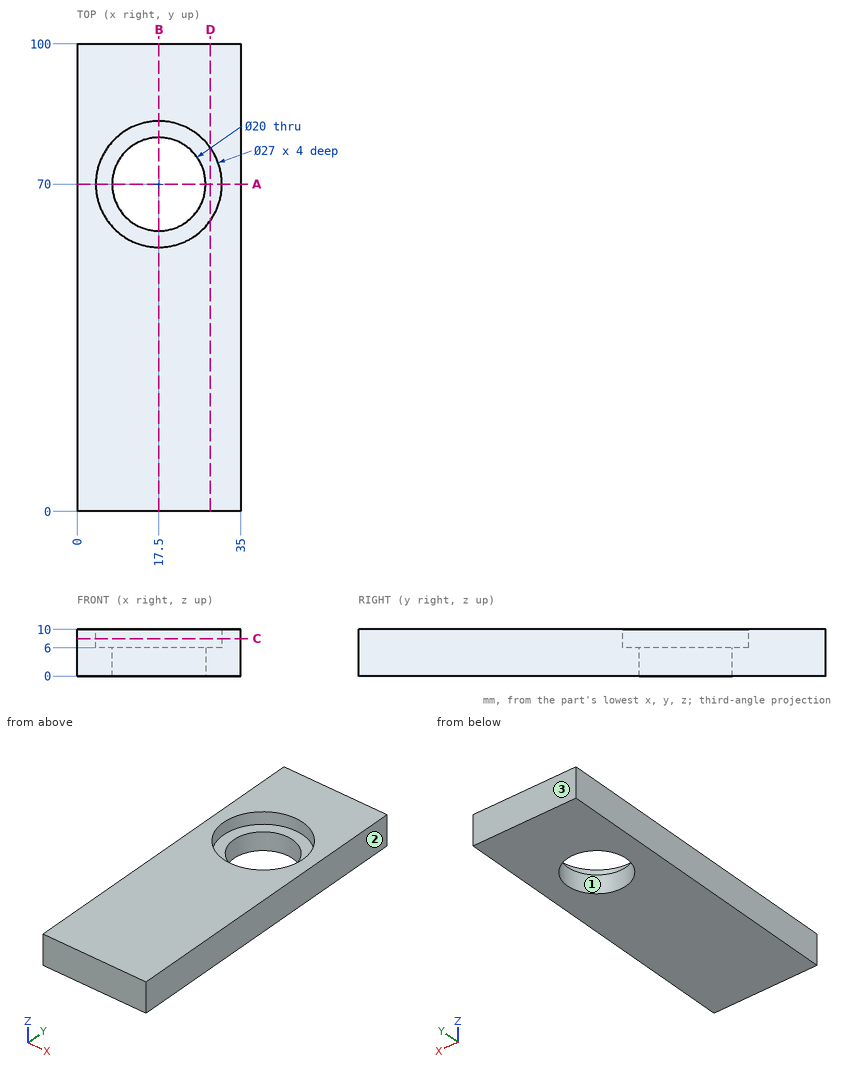
For this review, use the dimensioned drawing (mm, ordinates from the lowest corner) and the shaded views. Round coordinates to 2 decimals unless told otherwise and drop trailing zeros. Write each loop counter-clockwise with the first axis right and the second up, starting at its lowest first coordinate (ties: lowest second). Pieces come first, ordered by that corner, then holes. Notation, with made-up numbers: M 29.5,-33.5 L 82.5,-33.5 A11 cw 82.5,-27.5 Z; hole C 30.25,-20.5 d10. An arc over 180 degrees is marked long. Answer as CSV lines item,"result". Start each with the question number.
Q1. Consider section D-D, the plane x = 28.5. Give the boundary of the cut face in (y, z), then the cut area to 3 significant figures.
Q2. The part is to be moulded in two halves that separate along Y. For the marked faces 1, 2 and 3, say which applies: +Y half, -Y half, draft (parallel to the pull), parting line (faces both ways), or undercut.
Q3. Consider section B-B, the plane x = 17.5. Give the boundary of the cut face in (y, z).
Q4. Wall thickness on line 1 along Y through (x, z) = (17.5, 4); line 2 along Y through (x, z) = (17.5, 8.85); line 3 along Z through (x, y) = (4.5, 72.5): over which ranges is each line inside the solid? List them lowest first.
Q5. Consider section C-C, the plane z = 8. Give the boundary of the cut face in (x, y).
Q6. Consider section A-A, the plane y = 70. Give the boundary of the cut face in (x, z).
Result set:
1,outline,"M 0,0 L 100,0 L 100,10 L 77.83,10 L 77.83,6 L 62.17,6 L 62.17,10 L 0,10 Z"
1,area,"937 mm²"
2,face 1,"undercut"
2,face 2,"draft"
2,face 3,"+Y half"
3,outline,"M 0,0 L 60,0 L 60,6 L 56.5,6 L 56.5,10 L 0,10 Z; M 80,0 L 100,0 L 100,10 L 83.5,10 L 83.5,6 L 80,6 Z"
4,line 1,"y = 0 to 60, 80 to 100"
4,line 2,"y = 0 to 56.5, 83.5 to 100"
4,line 3,"z = 0 to 6"
5,outline,"M 0,0 L 35,0 L 35,100 L 0,100 Z; hole C 17.5,70 d27"
6,outline,"M 0,0 L 7.5,0 L 7.5,6 L 4,6 L 4,10 L 0,10 Z; M 27.5,0 L 35,0 L 35,10 L 31,10 L 31,6 L 27.5,6 Z"
